The figure shows three views and two pictorial views of one solid part (mm, origin at its lowest corner). Answer the questions. Coordinates: 2 decimals unless noted, no trailing zeros. Order: outer loops, then holes, each group sorted by start corner. A loop starts at its lowest first (then second) coordinate and runs counter-clockwise, first axis right, second up. Notation, with made-up numbers: (-21, 38) -> (-17, 38) arc R6 cw to (-17, 48) -> close; hole circle Ø1 at (40, 42). An arc over 180 degrees is marked (long way). Write item = value, one per line.
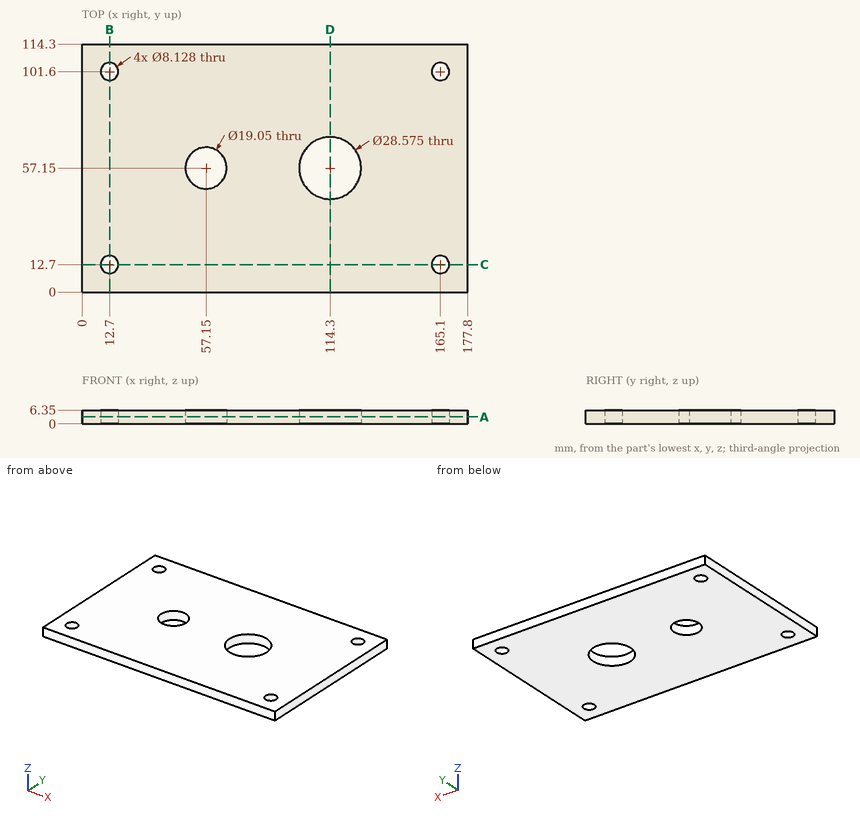
Q1. Section A-A, the plane z = 3.25 is taken. Give the number of separate pieces and of enclosed holes in the cut face, plus the area to 3 significant figures.
The answers:
separate_pieces = 1
enclosed_holes = 6
area = 19,200 mm2
Q2. Find the intervals of material crossed by line 1 along Y through (x, z) = (12.7, 2); line 2 along X through (y, z) = (56.5, 4.5); line 3 along X through (y, z) = (45.5, 0.5), in increasing order.
The answers:
line_1 = 0 to 8.64, 16.76 to 97.54, 105.66 to 114.3
line_2 = 0 to 47.65, 66.65 to 100.03, 128.57 to 177.8
line_3 = 0 to 106.03, 122.57 to 177.8
Q3. Section B-B, the plane x = 12.7 is taken. Give the vertices of the cut face in (y, z), plus the area to 3 significant figures.
The answers:
outline = (0, 0) -> (8.64, 0) -> (8.64, 6.35) -> (0, 6.35) -> close; (16.76, 0) -> (97.54, 0) -> (97.54, 6.35) -> (16.76, 6.35) -> close; (105.66, 0) -> (114.3, 0) -> (114.3, 6.35) -> (105.66, 6.35) -> close
area = 623 mm2
Q4. Section D-D, the plane x = 114.3 is taken. Give the vertices of the cut face in (y, z).
The answers:
outline = (0, 0) -> (42.86, 0) -> (42.86, 6.35) -> (0, 6.35) -> close; (71.44, 0) -> (114.3, 0) -> (114.3, 6.35) -> (71.44, 6.35) -> close
Q5. Section C-C, the plane y = 12.7 is taken. Give the vertices of the cut face in (x, z), plus the area to 3 significant figures.
The answers:
outline = (0, 0) -> (8.64, 0) -> (8.64, 6.35) -> (0, 6.35) -> close; (16.76, 0) -> (161.04, 0) -> (161.04, 6.35) -> (16.76, 6.35) -> close; (169.16, 0) -> (177.8, 0) -> (177.8, 6.35) -> (169.16, 6.35) -> close
area = 1,030 mm2
